For this review, use the dimensioned drawing (mm, ordinates from the lowest corner) and the shaded views. A direction names the side the tool comes from. Round coordinates to 2 decimals unless told otherwise and drop trailing zeros. Loops run counter-clockwise (first coordinate to the right, second up) from the corner with the lowest first, then second, coordinate; pieces in that order, holes last. Notation, with made-up numbers: (19.25, 77) - (63.25, 77) arc R27 ccw to (63.25, 94) - close; hole circle Ø9 at (27, -21.75). An arc over 180 degrees is marked (long way). Return JSON: item names as keys, results as strings. Group by question number.
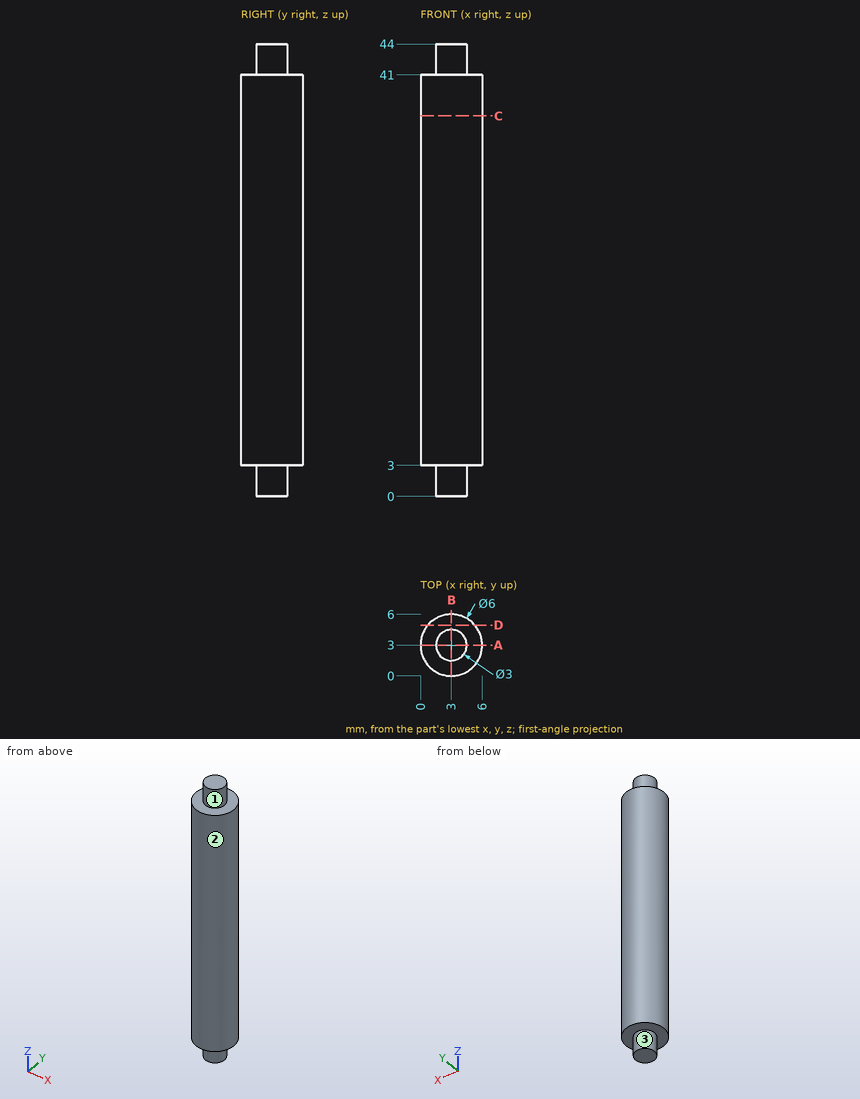
Q1. Add section C-C, the plane z = 37. State the section outline as (x, y) points, plus the area to 3 significant figures.
Q2. Add section A-A, the plane y = 3. State the section outline as (x, z) points.
Q3. Insertion check: pin 1 Ø1 at (x, y) = (3.5, 5) entering from -Z; pin 2 Ø3 at (y, z) = (5, 26.5) entering from -X; pin 3 Ø2 at (x, y) = (0.5, 3.5) entering from +Z. Each pin has a flat end and moves straight along its axis. Give the tip position at first contact, or say it passes through.
Q4. For line 1 (Z direction, x = 1.7, y = 4.1); line 2 (Y direction, x = 2.85, z = 15); line 3 (X direction, y = 1.95, z = 25), list the stretches that pass through material, from the lowest coordinate up.
Q5. Tool access review of the marked faces 1, 2 and 3: name each direction out of +Z, -Z, +X, -X, +Y, -Y from which nothing blocks a thin tool from reaching the whole face with its end or side.
Q6. Add section D-D, the plane y = 4.95. State the section outline as (x, z) points.
Evaluation:
{
 "1": {"outline": "circle Ø6 at (3, 3)", "area": "28.3 mm²"},
 "2": {"outline": "(0, 3) - (1.5, 3) - (1.5, 0) - (4.5, 0) - (4.5, 3) - (6, 3) - (6, 41) - (4.5, 41) - (4.5, 44) - (1.5, 44) - (1.5, 41) - (0, 41) - close"},
 "3": {"pin 1": "z = 3", "pin 2": "x = 0.04", "pin 3": "z = 41"},
 "4": {"line 1": "3 to 41", "line 2": "0 to 6", "line 3": "0.19 to 5.81"},
 "5": {"face 1": "+Z", "face 2": "+Z, -Z", "face 3": "-Z"},
 "6": {"outline": "(0.72, 3) - (5.28, 3) - (5.28, 41) - (0.72, 41) - close"}
}
